For this review, take the finished solid that the model builds, in its own axes (mm). A direction names the side the tool comes from. Coordinates: 2 decimals unless noted, no trailing zeros. Loops run counter-clockwise (first coordinate to the right, second up) from the corner with the lowest first, then second, coordinate; pieces in that order, holes last. Notation, with made-up numbers: (-26, 2.5) - (24, 2.5) arc R22 cw to (24, 41.5) - close; hole circle Ø7 at (63.25, 30). An arc over 180 degrees is marked (long way). Answer as a JSON object with one key per item and string values. Group by question number.
Item 1: Mouldability with a two-part tool opening along X and no side actions: class faces 1 (the flat face through (-31, 5, -48.25)), 2 (the flat face through (69, -34.081, 21)), 3 (the cylindrical face through (121.921, -1.004, 0.413)) as released by +X, released by -X, zero draft, split by the parting line, or undercut.
Item 2: We need section C-C (y = 81.5). Give the boundary of the cut face in (x, z), then the cut area to 3 significant figures.
Item 3: To check wall thickness, follow line 1 (X direction, y = 45.5, z = -8.5); line 2 (X direction, y = -3.5, z = -28); line 3 (X direction, y = 41, z = -27.5). State the ranges of each line that lie inside material, in increasing order.
Item 4: Tool access review of faces 4 (the flat face through (161.42, 57, -11)), 5 (the flat face through (181, 47, 20)), 6 (the cylindrical face through (80.953, 48.907, 0.035)), 7 (the cylindrical face through (54.41, -22.93, 21.64)), 8 (the flat face through (171.42, 47, 0)): name each direction out of +Z, -Z, +X, -X, +Y, -Y from which nothing blocks a thin tool from reaching the whole face with its end or side.
Item 5: We need section D-D (x = 19). Give the boundary of the cut face in (y, z).
Item 6: Clearance check with flat-ended pins moving along their axes: pin 1 (8 mm diameter, centred on x = 29, y = 33, fed in from +Z); pin 2 (20 mm diameter, centred on x = 130.5, z = 21.5, fed in from +Y); pin 3 (8 mm diameter, centred on x = 140.5, z = -9, fed in from -Y). State where each tip first meets the part, or that it passes through.
Item 7: We need section B-B (x = -11.5). Give the boundary of the cut face in (y, z), then the cut area to 3 significant figures.
Item 8: We need section A-A (z = -16.5). Give the boundary of the cut face in (x, y), then the cut area to 3 significant figures.
from build123d import *

# Parameters (mm, degrees)
SKETCH1_W                = 256.103174946
SKETCH1_H                = 133.5
BOSS_EXTRUDE1_DEPTH      = 48.25
SKETCH2_W                = 88
SKETCH2_H                = 45.5
CUT_EXTRUDE1_DEPTH       = 96.5
SKETCH4_W                = 39.103174946
SKETCH4_H                = 40
CUT_EXTRUDE2_DEPTH       = 96.5
SKETCH5_W                = 68
SKETCH5_H                = 76.5
CUT_EXTRUDE3_DEPTH       = 88
CUT_EXTRUDE4_DEPTH       = 133.5
CUT_EXTRUDE5_DEPTH       = 88
CUT_EXTRUDE6_DEPTH       = 88
SKETCH9_W                = 19.103174946
SKETCH9_H                = 20
CUT_EXTRUDE7_DEPTH       = 93.5
CUT_EXTRUDE8_DEPTH       = 73.5
CUT_EXTRUDE9_DEPTH       = 45.5
SKETCH17_W               = 46.042780748
SKETCH17_H               = 40
CUT_EXTRUDE12_DEPTH      = 40
CUT_EXTRUDE13_DEPTH      = 28
SKETCH23_W               = 40
SKETCH23_H               = 40
CUT_EXTRUDE20_DEPTH      = 8
SKETCH24_W               = 40
SKETCH24_H               = 40
CUT_EXTRUDE21_DEPTH      = 8
CUT_EXTRUDE22_DEPTH      = 14
CUT_EXTRUDE23_DEPTH      = 14
SKETCH29_R               = 5
CUT_EXTRUDE24_DEPTH      = 30
CUT_EXTRUDE24_DEPTH_BACK = 30
FILLET1_R                = 10
CUT_EXTRUDE25_DEPTH      = 26
CUT_EXTRUDE26_DEPTH      = 26
CUT_EXTRUDE28_DEPTH      = 40
CUT_EXTRUDE29_DEPTH      = 40
CUT_EXTRUDE30_DEPTH      = 40
CUT_EXTRUDE30_DEPTH_BACK = 40
FILLET2_R                = 10
FILLET3_R                = 10
FILLET4_R                = 10
CUT_EXTRUDE31_DEPTH      = 40
CUT_EXTRUDE31_DEPTH_BACK = 40
CUT_EXTRUDE32_DEPTH      = 2.5
CUT_EXTRUDE32_DEPTH_BACK = 2.5
SKETCH53_R               = 5
CUT_EXTRUDE33_DEPTH      = 43
CUT_EXTRUDE33_DEPTH_BACK = 43
BOSS_EXTRUDE4_DEPTH      = 2.5
BOSS_EXTRUDE4_DEPTH_BACK = 2.5
FILLET7_R                = 10


with BuildPart() as part:
    # Sketch1 → Boss-Extrude1 (new body, symmetric)
    with BuildSketch(Plane.XY):
        with Locations((72.471204682, 26.669157508)):
            Rectangle(SKETCH1_W, SKETCH1_H)
    extrude(amount=BOSS_EXTRUDE1_DEPTH, both=True)

    # Sketch2 → Cut-Extrude1 (cut)
    with BuildSketch(Plane.XY.offset(48.25)):
        with Locations((-11.580382791, 70.669157508)):
            Rectangle(SKETCH2_W, SKETCH2_H)
    extrude(amount=-CUT_EXTRUDE1_DEPTH, mode=Mode.SUBTRACT)

    # Sketch4 → Cut-Extrude2 (cut)
    with BuildSketch(Plane.XY.offset(48.25)):
        with Locations((180.971204682, -20.080842492)):
            Rectangle(SKETCH4_W, SKETCH4_H)
    extrude(amount=-CUT_EXTRUDE2_DEPTH, mode=Mode.SUBTRACT)

    # Sketch5 → Cut-Extrude3 (cut)
    with BuildSketch(Plane(origin=(0, 47.919157508, 0), x_dir=(1, 0, 0), z_dir=(0, 1, 0))):
        with Locations((-11.580382791, 0)):
            Rectangle(SKETCH5_W, SKETCH5_H)
    extrude(amount=-CUT_EXTRUDE3_DEPTH, mode=Mode.SUBTRACT)

    # Sketch6 → Cut-Extrude4 (cut)
    with BuildSketch(Plane(origin=(0, 93.419157508, 0), x_dir=(1, 0, 0), z_dir=(0, 1, 0))):
        Polygon((200.522792155, 48.25), (200.522792155, 20), (181.419617209, 20), (32.419617209, 42.509358289), (32.419617209, 48.25), align=None)
        Polygon((200.522792155, -48.25), (200.522792155, -20), (181.419617209, -20), (32.419617209, -42.509358289), (32.419617209, -48.25), align=None)
    extrude(amount=-CUT_EXTRUDE4_DEPTH, mode=Mode.SUBTRACT)

    # Sketch7 → Cut-Extrude5 (cut)
    with BuildSketch(Plane(origin=(0, 47.919157508, 0), x_dir=(1, 0, 0), z_dir=(0, 1, 0))):
        Polygon((-5.580382791, 48.25), (32.419617209, 42.509358289), (32.419617209, 48.25), align=None)
    extrude(amount=-CUT_EXTRUDE5_DEPTH, mode=Mode.SUBTRACT)

    # Sketch8 → Cut-Extrude6 (cut)
    with BuildSketch(Plane(origin=(0, 47.919157508, 0), x_dir=(1, 0, 0), z_dir=(0, 1, 0))):
        Polygon((-5.580382791, -48.25), (32.419617209, -42.509358289), (32.419617209, -48.25), align=None)
    extrude(amount=-CUT_EXTRUDE6_DEPTH, mode=Mode.SUBTRACT)

    # Sketch9 → Cut-Extrude7 (cut)
    with BuildSketch(Plane(origin=(0, 93.419157508, 0), x_dir=(1, 0, 0), z_dir=(0, 1, 0))):
        with Locations((180.971204682, 0)):
            Rectangle(SKETCH9_W, SKETCH9_H)
    extrude(amount=-CUT_EXTRUDE7_DEPTH, mode=Mode.SUBTRACT)

    # Sketch10 → Cut-Extrude8 (cut)
    with BuildSketch(Plane(origin=(0, 93.419157508, 0), x_dir=(1, 0, 0), z_dir=(0, 1, 0))):
        Polygon((161.419617209, 20), (181.419617209, 20), (161.419617209, 23.021390374), align=None)
        Polygon((181.419617209, -20), (161.419617209, -20), (161.419617209, -23.021390374), align=None)
    extrude(amount=-CUT_EXTRUDE8_DEPTH, mode=Mode.SUBTRACT)

    # Sketch14 → Cut-Extrude9 (cut)
    with BuildSketch(Plane(origin=(0, 93.419157508, 0), x_dir=(1, 0, 0), z_dir=(0, 1, 0))):
        Polygon((161.419617209, 20), (161.419617209, 2.5), (32.419617209, 2.5), (32.419617209, 42.509358289), (161.419617209, 23.021390374), align=None)
        Polygon((161.419617209, -20), (161.419617209, -2.5), (32.419617209, -2.5), (32.419617209, -42.509358289), (161.419617209, -23.021390374), align=None)
    extrude(amount=-CUT_EXTRUDE9_DEPTH, mode=Mode.SUBTRACT)

    # Sketch17 → Cut-Extrude12 (cut)
    with BuildSketch(Plane(origin=(161.419617209, 0, 0), x_dir=(0, 0, -1), z_dir=(1, 0, 0))):
        with Locations((0, -20.080842492)):
            Rectangle(SKETCH17_W, SKETCH17_H)
    extrude(amount=-CUT_EXTRUDE12_DEPTH, mode=Mode.SUBTRACT)

    # Sketch19 → Cut-Extrude13 (cut)
    with BuildSketch(Plane(origin=(0, 47.919157508, 0), x_dir=(1, 0, 0), z_dir=(0, 1, 0))):
        Polygon((32.419617209, -2.5), (32.419617209, -42.509358289), (161.419617209, -23.021390374), (161.419617209, -20), (161.419617209, -2.5), align=None)
        Polygon((32.419617209, 2.5), (32.419617209, 42.509358289), (161.419617209, 23.021390374), (161.419617209, 2.5), align=None)
    extrude(amount=-CUT_EXTRUDE13_DEPTH, mode=Mode.SUBTRACT)

    # Sketch23 → Cut-Extrude20 (cut)
    with BuildSketch(Plane(origin=(0, 0, 23.021390374), x_dir=(-1, 0, 0), z_dir=(0, 0, -1))):
        with Locations((-141.419617209, -20.080842492)):
            Rectangle(SKETCH23_W, SKETCH23_H)
    extrude(amount=-CUT_EXTRUDE20_DEPTH, mode=Mode.SUBTRACT)

    # Sketch24 → Cut-Extrude21 (cut)
    with BuildSketch(Plane.XY.offset(-23.021390374)):
        with Locations((141.419617209, -20.080842492)):
            Rectangle(SKETCH24_W, SKETCH24_H)
    extrude(amount=-CUT_EXTRUDE21_DEPTH, mode=Mode.SUBTRACT)

    # Sketch26 → Cut-Extrude22 (cut)
    with BuildSketch(Plane(origin=(0, 19.919157508, 0), x_dir=(1, 0, 0), z_dir=(0, 1, 0))):
        Polygon((141.419617209, -2.5), (141.419617209, -26.042780749), (32.419617209, -42.509358289), (32.419617209, -2.5), align=None)
    extrude(amount=-CUT_EXTRUDE22_DEPTH, mode=Mode.SUBTRACT)

    # Sketch27 → Cut-Extrude23 (cut)
    with BuildSketch(Plane(origin=(0, 19.919157508, 0), x_dir=(1, 0, 0), z_dir=(0, 1, 0))):
        Polygon((141.419617209, 2.5), (32.419617209, 2.5), (32.419617209, 42.509358289), (141.419617209, 26.042780749), align=None)
    extrude(amount=-CUT_EXTRUDE23_DEPTH, mode=Mode.SUBTRACT)

    # Sketch29 → Cut-Extrude24 (cut, two sides)
    with BuildSketch(Plane.XY) as cut_extrude24_sk:
        with Locations((151.419617209, 9.919157508)):
            Circle(SKETCH29_R)
    extrude(amount=CUT_EXTRUDE24_DEPTH, mode=Mode.SUBTRACT)
    extrude(cut_extrude24_sk.sketch, amount=-CUT_EXTRUDE24_DEPTH_BACK, mode=Mode.SUBTRACT)

    # Fillet1
    fillet1_edges = [part.edges().sort_by_distance(p)[0] for p in [
        (141.419617209, 19.919157508, 14.271390374),
    ]]
    fillet(fillet1_edges, radius=FILLET1_R)

    # Sketch31 → Cut-Extrude25 (cut)
    with BuildSketch(Plane(origin=(0, 5.919157508, 0), x_dir=(1, 0, 0), z_dir=(0, 1, 0))):
        Polygon((32.419617209, -2.5), (57.419617209, -2.5), (57.419617209, -38.732620321), (32.419617209, -42.509358289), align=None)
    extrude(amount=-CUT_EXTRUDE25_DEPTH, mode=Mode.SUBTRACT)

    # Sketch32 → Cut-Extrude26 (cut)
    with BuildSketch(Plane(origin=(0, 5.919157508, 0), x_dir=(1, 0, 0), z_dir=(0, 1, 0))):
        Polygon((32.419617209, 2.5), (57.419617209, 2.5), (57.419617209, 38.732620321), (32.419617209, 42.509358289), align=None)
    extrude(amount=-CUT_EXTRUDE26_DEPTH, mode=Mode.SUBTRACT)

    # Sketch40 → Cut-Extrude28 (cut)
    with BuildSketch(Plane(origin=(0, 5.919157508, 0), x_dir=(1, 0, 0), z_dir=(0, 1, 0))):
        Polygon((57.419617209, 38.732620321), (81.352447073, 35.117099232), (81.352447073, 2.5), (57.419617209, 2.5), align=None)
    extrude(amount=-CUT_EXTRUDE28_DEPTH, mode=Mode.SUBTRACT)

    # Sketch41 → Cut-Extrude29 (cut)
    with BuildSketch(Plane(origin=(0, 5.919157508, 0), x_dir=(1, 0, 0), z_dir=(0, 1, 0))):
        Polygon((57.419617209, -2.5), (57.419617209, -38.732620321), (81.352447073, -35.117099232), (81.352447073, -2.5), align=None)
    extrude(amount=-CUT_EXTRUDE29_DEPTH, mode=Mode.SUBTRACT)

    # Sketch43 → Cut-Extrude30 (cut, two sides)
    with BuildSketch(Plane.XY) as cut_extrude30_sk:
        Polygon((88.23219723, -40.080842492), (121.419617209, -0.080842492), (121.419617209, -40.080842492), align=None)
    extrude(amount=CUT_EXTRUDE30_DEPTH, mode=Mode.SUBTRACT)
    extrude(cut_extrude30_sk.sketch, amount=-CUT_EXTRUDE30_DEPTH_BACK, mode=Mode.SUBTRACT)

    # Fillet2
    fillet2_edges = [part.edges().sort_by_distance(p)[0] for p in [
        (121.419617209, -0.080842492, 0),
        (88.23219723, -40.080842492, 0),
    ]]
    fillet(fillet2_edges, radius=FILLET2_R)

    # Fillet3
    fillet3_edges = [part.edges().sort_by_distance(p)[0] for p in [
        (57.419617209, -20.080842492, 20.61631016),
    ]]
    fillet(fillet3_edges, radius=FILLET3_R)

    # Fillet4
    fillet4_edges = [part.edges().sort_by_distance(p)[0] for p in [
        (57.419617209, -20.080842492, -20.61631016),
    ]]
    fillet(fillet4_edges, radius=FILLET4_R)

    # Sketch44 → Cut-Extrude31 (cut, two sides)
    with BuildSketch(Plane.XY) as cut_extrude31_sk:
        Polygon((81.352447073, 5.919157508), (118.653161204, 5.919157508), (85.465741224, -34.080842492), (81.352447073, -34.080842492), align=None)
    extrude(amount=CUT_EXTRUDE31_DEPTH, mode=Mode.SUBTRACT)
    extrude(cut_extrude31_sk.sketch, amount=-CUT_EXTRUDE31_DEPTH_BACK, mode=Mode.SUBTRACT)

    # Sketch49 → Cut-Extrude32 (cut, two sides)
    with BuildSketch(Plane.XY) as cut_extrude32_sk:
        Polygon((118.653161204, 5.919157508), (118.653161204, 93.419157508), (32.419617209, 93.419157508), (32.419617209, 47.919157508), (81.352447073, 47.919157508), (81.352447073, 5.919157508), align=None)
    extrude(amount=CUT_EXTRUDE32_DEPTH, mode=Mode.SUBTRACT)
    extrude(cut_extrude32_sk.sketch, amount=-CUT_EXTRUDE32_DEPTH_BACK, mode=Mode.SUBTRACT)

    # Sketch53 → Cut-Extrude33 (cut, two sides)
    with BuildSketch(Plane.XY) as cut_extrude33_sk:
        with Locations((47.419617209, -30.080842492)):
            Circle(SKETCH53_R)
    extrude(amount=CUT_EXTRUDE33_DEPTH, mode=Mode.SUBTRACT)
    extrude(cut_extrude33_sk.sketch, amount=-CUT_EXTRUDE33_DEPTH_BACK, mode=Mode.SUBTRACT)

    # Sketch55 → Boss-Extrude4 (add, two sides)
    with BuildSketch(Plane.XY) as boss_extrude4_sk:
        Polygon((81.352447073, 47.919157508), (118.653161204, 93.419157508), (118.653161204, 5.919157508), (85.465741224, -34.080842492), (80.854981216, -34.080842492), align=None)
    extrude(amount=BOSS_EXTRUDE4_DEPTH)
    extrude(boss_extrude4_sk.sketch, amount=-BOSS_EXTRUDE4_DEPTH_BACK)

    # Fillet7
    fillet7_edges = [part.edges().sort_by_distance(p)[0] for p in [
        (141.419617209, 19.919157508, -14.271390374),
        (85.465741224, -34.080842492, 18.497852932),
        (118.653161204, 5.919157508, 15.99104915),
        (118.653161204, 5.919157508, -15.99104915),
        (118.653161204, 93.419157508, 0),
        (81.352447073, 47.919157508, 0),
        (85.465741224, -34.080842492, -18.497852932),
    ]]
    fillet(fillet7_edges, radius=FILLET7_R)


solid = part.part
Check sheet entries:
{
 "1": {"face 1": "zero draft", "face 2": "undercut", "face 3": "released by +X"},
 "2": {"outline": "(108.88, -2.5) - (161.42, -2.5) - (161.42, -20) - (200.52, -20) - (200.52, 20) - (161.42, 20) - (161.42, 2.5) - (108.88, 2.5) - close; hole (171.42, -10) - (190.52, -10) - (190.52, 10) - (171.42, 10) - close", "area": "1,440 mm2"},
 "3": {"line 1": "x = -55.58 to -45.58, 22.42 to 32.42, 161.42 to 171.42, 190.52 to 200.52", "line 2": "x = -55.58 to -45.58, 22.42 to 32.42, 110.84 to 118.59", "line 3": "x = -55.58 to -45.58, 22.42 to 32.42"},
 "4": {"face 4": "-Z, +Y", "face 5": "+Z, +X, +Y", "face 6": "+Z, -Z, -X, +Y", "face 7": "+Z, +Y", "face 8": "+Y, -Y"},
 "5": {"outline": "(-40.08, -44.54) - (47.92, -44.54) - (47.92, -38.25) - (-40.08, -38.25) - close; (-40.08, 38.25) - (47.92, 38.25) - (47.92, 44.54) - (-40.08, 44.54) - close"},
 "6": {"pin 1": "stops at z = 43.63", "pin 2": "stops at y = 5.92", "pin 3": "stops at y = -0.08"},
 "7": {"outline": "(-40.08, -48.25) - (47.92, -48.25) - (47.92, -38.25) - (-40.08, -38.25) - close; (-40.08, 38.25) - (47.92, 38.25) - (47.92, 48.25) - (-40.08, 48.25) - close", "area": "1,760 mm2"},
 "8": {"outline": "(-55.58, -40.08) - (-45.58, -40.08) - (-45.58, 47.92) - (-55.58, 47.92) - close; (22.42, -40.08) - (83.54, -40.08) arc R10 ccw to (91.23, -36.47) - (118.42, -3.7) arc R10 cw to (126.12, -0.08) - (200.52, -0.08) - (200.52, 93.42) - (161.42, 93.42) - (161.42, 19.92) - (151.42, 19.92) arc R10 ccw to (141.42, 9.92) - (141.42, 5.92) - (123.35, 5.92) arc R10 ccw to (115.65, 2.3) - (88.46, -30.47) arc R10 cw to (80.77, -34.08) - (57.42, -34.08) - (57.42, -30.08) arc R10 ccw to (47.42, -20.08) - (32.42, -20.08) - (32.42, 47.92) - (22.42, 47.92) - close; hole circle Ø10 at (47.42, -30.08); hole circle Ø10 at (151.42, 9.92)", "area": "6,730 mm2"}
}
